CAD build for the part. Positions are in the model's coordinates, mm. Face numbers are marked on the shaded views. A direction names the side the tool comes from. Give positions to 0.01 mm unless a question says otherwise; leave off trailing zeros. Write each loop counter-clockwise with the first axis right and the second up, starting at its lowest first coordinate (ties: lowest second). Pieces come first, ordered by that corner, then holes. Notation, with made-up numbers: (82.5, 42) -> (124.5, 42) arc R11 ccw to (124.5, 63) -> close; hole circle Ø3 at (-39.75, 52). An arc over 180 degrees is marked (long way). Answer as a JSON object with one key per item and string values.
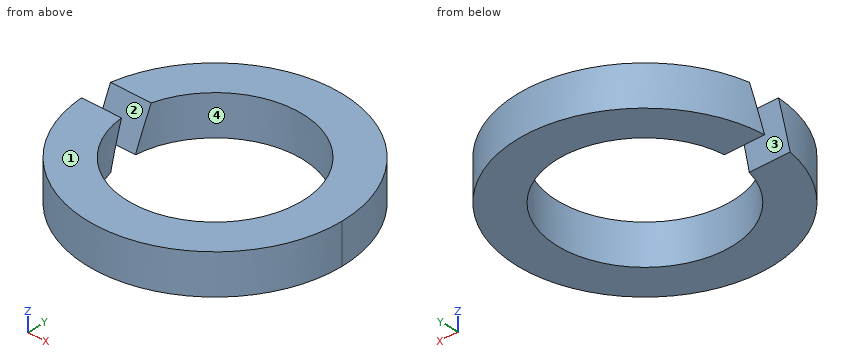
```python
from build123d import *

# Parameters (mm, degrees)
SKETCH_1_R          = 4.45
SKETCH_1_R_2        = 3.05
EXTRUDE_1_DEPTH     = 1.4
CUT_EXTRUDE_1_DEPTH = 7.447092368


with BuildPart() as part:
    # Эскиз1 → Вытянуть1 (new body)
    with BuildSketch(Plane.XY):
        Circle(SKETCH_1_R)
        Circle(SKETCH_1_R_2, mode=Mode.SUBTRACT)
    extrude(amount=EXTRUDE_1_DEPTH)

    # Эскиз2 → Вырез-Вытянуть1 (cut, through all)
    with BuildSketch(Plane(origin=(0, 0, 0), x_dir=(0, 0, -1), z_dir=(1, 0, 0))):
        Polygon((0, 0.266667945), (-1.4, 0.776226272), (-1.4, 0), (-1.4, -0.266667945), (0, -0.776226272), (0, 0), align=None)
    extrude(amount=-CUT_EXTRUDE_1_DEPTH, mode=Mode.SUBTRACT)


solid = part.part
```
1) Slice it at B-B (y = -1.25). List the corners of the cut face in (x, z), then the cut area to 3 significant figures.
Model answer:
{"outline": "(-4.27, 0) -> (-2.78, 0) -> (-2.78, 1.4) -> (-4.27, 1.4) -> close; (2.78, 0) -> (4.27, 0) -> (4.27, 1.4) -> (2.78, 1.4) -> close", "area": "4.17 mm2"}
2) Mould opens along Y. For the marked faces 1 and 2 say: released by +Y, released by -Y, zero draft, split by the parting line, or undercut.
Model answer:
{"face 1": "zero draft", "face 2": "undercut"}
3) Slice it at C-C (z = 1.15). List the corners of the cut face in (x, y).
Model answer:
{"outline": "(-4.44, -0.36) arc R4.45 ccw (long way) to (-4.4, 0.69) -> (-2.97, 0.69) arc R3.05 cw (long way) to (-3.03, -0.36) -> close"}
4) Slice it at A-A (x = 0). List the corners of the cut face in (y, z), then the cut area to 3 significant figures.
Model answer:
{"outline": "(-4.45, 0) -> (-3.05, 0) -> (-3.05, 1.4) -> (-4.45, 1.4) -> close; (3.05, 0) -> (4.45, 0) -> (4.45, 1.4) -> (3.05, 1.4) -> close", "area": "3.92 mm2"}
5) Wall check: probe 1 along Y at (x, z) = (0, 0.5); probe 2 along X at (y, z) = (0, 1.05); probe 3 along Y at (x, z) = (-4, 0.85). Give the ranges that are in metal, low to high.
Model answer:
{"probe 1": "y = -4.45 to -3.05, 3.05 to 4.45", "probe 2": "x = 3.05 to 4.45", "probe 3": "y = -1.95 to -0.47, 0.58 to 1.95"}
6) 3-axis set-ups, long thin cutter, end or side, ignore diameter. For the marked faces 3 and 4: which of +Z, -Z, +X, -X, +Y, -Y reach the whole face in a straight line?
Model answer:
{"face 3": "-Z, -X", "face 4": "+Z, -Z"}
